from build123d import *

# Parameters (mm, degrees)
SKETCH1_R           = 69.85
SKETCH1_R_2         = 9.525
BOSS_EXTRUDE1_DEPTH = 3.175
SKETCH2_R           = 8.001
SKETCH2_R_2         = 3.556
CUT_EXTRUDE1_DEPTH  = 3.175
SKETCH3_R           = 1.750000056
SKETCH3_R_2         = 1.75
CUT_EXTRUDE2_DEPTH  = 50.8


with BuildPart() as part:
    # Sketch1 → Boss-Extrude1 (new body)
    with BuildSketch(Plane(origin=(0, 0, 0), x_dir=(1, 0, 0), z_dir=(0, 1, 0))):
        with Locations(Location((0, 0, 0), (0, 0, 270))):
            Circle(SKETCH1_R)
        with Locations(Location((0, 0, 0), (0, 0, 270))):
            Circle(SKETCH1_R_2, mode=Mode.SUBTRACT)
    extrude(amount=BOSS_EXTRUDE1_DEPTH)

    # Sketch2 → Cut-Extrude1 (cut)
    with BuildSketch(Plane(origin=(0, 3.175, 0), x_dir=(1, 0, 0), z_dir=(0, 1, 0))):
        with Locations(Location((-59.69, 0, 0), (0, 0, 270))):
            Circle(SKETCH2_R)
        with Locations(Location((59.69, 0, 0), (0, 0, 270))):
            Circle(SKETCH2_R)
        with Locations(Location((-51.795490029, -24.152633658, 0), (0, 0, 270))):
            Circle(SKETCH2_R_2)
        with Locations(Location((51.795490029, 24.152633658, 0), (0, 0, 270))):
            Circle(SKETCH2_R_2)
    extrude(amount=-CUT_EXTRUDE1_DEPTH, mode=Mode.SUBTRACT)

    # Sketch3 → Cut-Extrude2 (cut)
    with BuildSketch(Plane(origin=(0, 3.175, 0), x_dir=(1, 0, 0), z_dir=(0, 1, 0))):
        with Locations(Location((15.5, 15.5, 0), (0, 0, 270))):
            Circle(SKETCH3_R)
        with Locations(Location((15.5, -15.5, 0), (0, 0, 270))):
            Circle(SKETCH3_R)
        with Locations(Location((-15.5, -15.5, 0), (0, 0, 270))):
            Circle(SKETCH3_R)
        with Locations(Location((-15.5, 15.5, 0), (0, 0, 270))):
            Circle(SKETCH3_R_2)
    extrude(amount=-CUT_EXTRUDE2_DEPTH, mode=Mode.SUBTRACT)


solid = part.part
The listing builds one solid part. Answer for the finished solid, in the listing's coordinates (mm). Give positions to 0.01 mm unless a question says otherwise; leave off trailing zeros. Loops run counter-clockwise (first coordinate to the right, second up) from the corner with the lowest first, then second, coordinate; pieces in that order, holes last. Notation, with made-up numbers: M 68,-3.5 L 105,-3.5 A11 ccw 105,8.5 Z; hole C 39.5,27.25 d11. An arc over 180 degrees is marked long. Answer as CSV lines item,"result".
Item 1: The mould has two halves that part along Z. Classify faces 1 (the cylindrical face through (-51.757, 1.61, -1.042)), 2 (the flat face through (1, 3.175, 15)), 3 (the cylindrical face through (-68.2, 1.6, -15.1)): released by +Z, released by -Z, zero draft, split by the parting line, or undercut.
Values follow:
face 1,"undercut"
face 2,"zero draft"
face 3,"split by the parting line"
Item 2: Given pin 1 Ø1 at (x, y) = (-45, 0.5) entering from +Z; pin 2 Ø1 at (y, z) = (2, -52) entering from +X, each flat-ended and moving along its own axis, determine where each tip first touches the part or whether it passes through.
Values follow:
pin 1,"stops at z = 53.84"
pin 2,"stops at x = 47.19"
Item 3: Straight lines are drawn through the part: line 1 along X through (y, z) = (0.7, 0) (3 decimals); line 2 along X through (y, z) = (0.35, -17); line 3 along X through (y, z) = (0.75, -2.5). For each, find the intervals that lie inside material, in ascending order. Write a range as [from, to].
Values follow:
line 1,"x = [-69.85, -67.691], [-51.689, -9.525], [9.525, 51.689], [67.691, 69.85]"
line 2,"x = [-67.75, -16.4], [-14.6, 14.6], [16.4, 67.75]"
line 3,"x = [-69.81, -67.29], [-52.09, -9.19], [9.19, 52.09], [67.29, 69.81]"
Item 4: The part is cut by section D-D (z = -15.5). Give the vertices of the cut face in (x, y) (3 decimals).
Values follow:
outline,"M -68.109,0 L -17.25,0 L -17.25,3.175 L -68.109,3.175 Z; M -13.75,0 L 13.75,0 L 13.75,3.175 L -13.75,3.175 Z; M 17.25,0 L 68.109,0 L 68.109,3.175 L 17.25,3.175 Z"
Item 5: The part is cut by section B-B (z = 0). Give the vertices of the cut face in (x, y) (3 decimals).
Values follow:
outline,"M -69.85,0 L -67.691,0 L -67.691,3.175 L -69.85,3.175 Z; M -51.689,0 L -9.525,0 L -9.525,3.175 L -51.689,3.175 Z; M 9.525,0 L 51.689,0 L 51.689,3.175 L 9.525,3.175 Z; M 67.691,0 L 69.85,0 L 69.85,3.175 L 67.691,3.175 Z"
Item 6: The part is cut by section A-A (x = 0). Give the vertices of the cut face in (y, z) (3 decimals), and give its area (3 significant figures).
Values follow:
outline,"M 0,-69.85 L 3.175,-69.85 L 3.175,-9.525 L 0,-9.525 Z; M 0,9.525 L 3.175,9.525 L 3.175,69.85 L 0,69.85 Z"
area,"383 mm^2"
Item 7: The part is cut by section C-C (x = -15.5). Give the vertices of the cut face in (y, z) (3 decimals).
Values follow:
outline,"M 0,-68.109 L 3.175,-68.109 L 3.175,-17.25 L 0,-17.25 Z; M 0,-13.75 L 3.175,-13.75 L 3.175,13.75 L 0,13.75 Z; M 0,17.25 L 3.175,17.25 L 3.175,68.109 L 0,68.109 Z"
